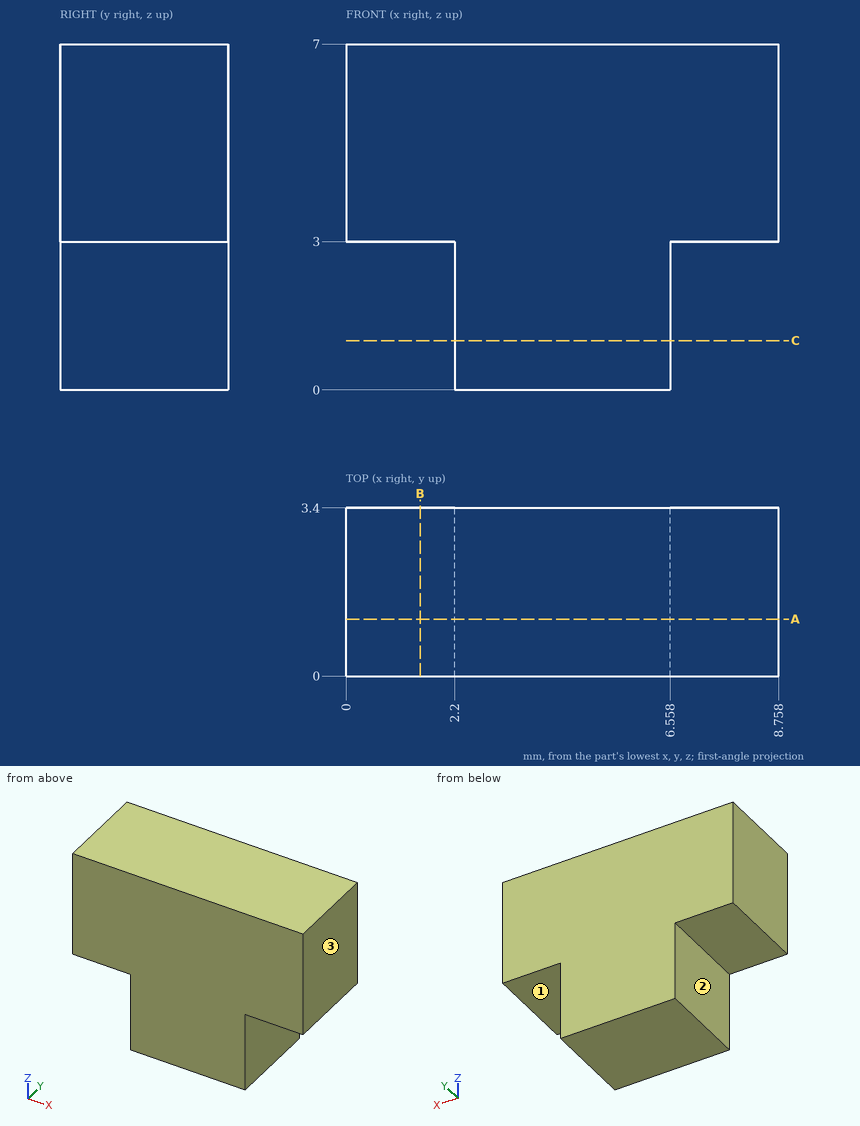
Answer from the drawing. Dimensions are ordinates in mm from the lowest x, y and z of the part. A direction names the side the tool comes from. Coordinates: 2 decimals unless noted, no trailing zeros. Write each loop counter-clockwise with the first axis right and the second up, starting at its lowest first coordinate (ties: lowest second). Pieces come first, ordered by that corner, then holes. Notation, with made-up numbers: (88.25, 0.25) -> (121.25, 0.25) arc R18 ccw to (121.25, 8.25) -> close; hole circle Ø6 at (23.5, 21.25). An arc over 180 degrees is marked (long way). One line per question, with ' | ' between items.
1. Section C-C (z = 1) is taken. Determine the outline of the cut face in (x, y), and give its area (3 significant figures).
Verdict:
outline: (2.2, 0) -> (6.56, 0) -> (6.56, 3.4) -> (2.2, 3.4) -> close | area: 14.8 mm^2
2. Section B-B (x = 1.5) is taken. Determine the outline of the cut face in (y, z).
Verdict:
outline: (0, 3) -> (3.4, 3) -> (3.4, 7) -> (0, 7) -> close
3. Section A-A (y = 1.15) is taken. Determine the outline of the cut face in (x, z), and give its area (3 significant figures).
Verdict:
outline: (0, 3) -> (2.2, 3) -> (2.2, 0) -> (6.56, 0) -> (6.56, 3) -> (8.76, 3) -> (8.76, 7) -> (0, 7) -> close | area: 48.1 mm^2
4. Given pin 1 Ø0.9 at (y, z) = (1, 1) entering from -X; pin 2 Ø1 at (y, z) = (1.5, 6) entering from -X; pin 3 Ø1.8 at (x, y) = (1, 1.5) entering from -Z; pin 4 Ø2 at (y, z) = (0.5, 1.5) entering from +X, each flat-ended and moving along its own axis, determine where each tip first touches the part or whether it passes through.
Verdict:
pin 1: stops at x = 2.2 | pin 2: stops at x = 0 | pin 3: stops at z = 3 | pin 4: stops at x = 6.56
5. Straight lines are drawn through the part: line 1 (X direction, y = 0.95, z = 1.5); line 2 (Z direction, x = 7, y = 1.6). For each, find the intervals that lie inside material, in ascending order.
Verdict:
line 1: x = 2.2 to 6.56 | line 2: z = 3 to 7
6. Which of the six approach directions +Z, -Z, +X, -X, +Y, -Y give full straight-line access (tool end or side, diameter ignored) to the marked faces 1, 2 and 3?
Verdict:
face 1: -Z, +X, +Y, -Y | face 2: -Z, -X, +Y, -Y | face 3: +Z, -Z, +X, +Y, -Y
